Verification items for the finished model (mm, model axes). Coordinates: 2 decimals unless noted, no trailing zeros. Order: outer loops, then holes, each group sorted by start corner. A loop starts at its lowest first (then second) coordinate and runs counter-clockwise, first axis right, second up.
Q1. Cross-section at C-C, the plane z = 75.5. Record the boundary of the cut face in (x, y).
Q2. Cross-section at A-A, the plane x = 0. Record the boundary of the cut face in (y, z) (3 decimals).
Q3. Depth check by flat-ended pin: P1, Ø2.5, axis at x = 1.5, y = -0.5, coming from the +Z side; P2, Ø2, axis at x = -2, z = 18, coming from the -Y side; P3, Ø3, axis at x = 0, y = 0, coming from the -Z side; P4, Ø3, axis at x = 0, y = 1, coming from the -Z side. Enter the tip coordinate at first touch or a pass-through.
Q4. Thickness scan on line 1 (X direction, y = 0.25, z = 63); line 2 (Y direction, x = 0, z = 0.9); line 3 (Z direction, x = -2.75, y = 1.5). Record the ranges inside material, lowest first.
from build123d import *

# Parameters (mm, degrees)
SKETCH1_R           = 5.5
SKETCH1_R_2         = 2.025
BOSS_EXTRUDE1_DEPTH = 92.5
SKETCH2_R           = 4.5
CUT_EXTRUDE1_DEPTH  = 2
SKETCH3_R           = 4.5
CUT_EXTRUDE2_DEPTH  = 2
SKETCH4_R           = 3
CUT_EXTRUDE3_DEPTH  = 43


with BuildPart() as part:
    # Sketch1 → Boss-Extrude1 (new body)
    with BuildSketch(Plane.XY):
        Circle(SKETCH1_R)
        Circle(SKETCH1_R_2, mode=Mode.SUBTRACT)
    extrude(amount=BOSS_EXTRUDE1_DEPTH)

    # Sketch2 → Cut-Extrude1 (cut)
    with BuildSketch(Plane.XY.offset(92.5)):
        Circle(SKETCH2_R)
    extrude(amount=-CUT_EXTRUDE1_DEPTH, mode=Mode.SUBTRACT)

    # Sketch3 → Cut-Extrude2 (cut)
    with BuildSketch(Plane(origin=(0, 0, 0), x_dir=(-1, 0, 0), z_dir=(0, 0, -1))):
        Circle(SKETCH3_R)
    extrude(amount=-CUT_EXTRUDE2_DEPTH, mode=Mode.SUBTRACT)

    # Sketch4 → Cut-Extrude3 (cut, symmetric)
    with BuildSketch(Plane.XY.offset(46.25)):
        Circle(SKETCH4_R)
    extrude(amount=CUT_EXTRUDE3_DEPTH, both=True, mode=Mode.SUBTRACT)


solid = part.part
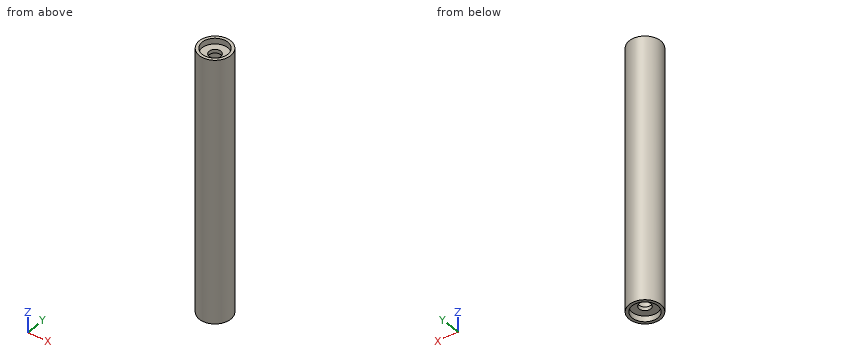
Check values:
1. outline: circle Ø11 at (0, 0); hole circle Ø6 at (0, 0)
2. outline: (-5.5, 0) - (-4.5, 0) - (-4.5, 2) - (-2.025, 2) - (-2.025, 3.25) - (-3, 3.25) - (-3, 89.25) - (-2.025, 89.25) - (-2.025, 90.5) - (-4.5, 90.5) - (-4.5, 92.5) - (-5.5, 92.5) - close; (2.025, 2) - (4.5, 2) - (4.5, 0) - (5.5, 0) - (5.5, 92.5) - (4.5, 92.5) - (4.5, 90.5) - (2.025, 90.5) - (2.025, 89.25) - (3, 89.25) - (3, 3.25) - (2.025, 3.25) - close
3. P1: stops at z = 90.5
3. P2: stops at y = -5.41
3. P3: passes through
3. P4: stops at z = 2
4. line 1: x = -5.49 to -2.99, 2.99 to 5.49
4. line 2: y = -5.5 to -4.5, 4.5 to 5.5
4. line 3: z = 2 to 90.5
